from build123d import *

# Parameters (mm, degrees)
F0_W     = 1.5
F0_H     = 30
F1_DEPTH = 3
F0_H_2   = 5
F2_DEPTH = 20
F0_H_3   = 3
F3_DEPTH = 110


with BuildPart() as f1:
    # F0 (on Top) → F1 (new body)
    with BuildSketch(Plane.XY):
        Polygon((12.5, -5), (12.5, 30), (0.75, 30), (0.75, 0), (-0.75, 0), (-0.75, 30), (-12.5, 30), (-12.5, -5), (0, -5), align=None)
        with Locations((0, 15)):
            Rectangle(F0_W, F0_H)
        Polygon((0, -30), (0, -5), (-12.5, -5), (-12.5, -17.5), align=None)
        Polygon((12.5, -17.5), (12.5, -5), (0, -5), (0, -30), align=None)
        Polygon((25, -5), (12.5, -5), (12.5, -17.5), align=None)
        Polygon((-12.5, -17.5), (-12.5, -5), (-25, -5), align=None)
    extrude(amount=F1_DEPTH)

    # F0 (on Top) → F2 (join)
    with BuildSketch(Plane.XY):
        with Locations((0, 32.5)):
            Rectangle(F0_W, F0_H_2)
        with Locations((0, 15)):
            Rectangle(F0_W, F0_H)
        Polygon((0.75, 35), (0.75, 30), (4.75, 35), align=None)
        Polygon((-4.75, 35), (-0.75, 30), (-0.75, 35), align=None)
    extrude(amount=F2_DEPTH)

    # F0 (on Top) → F3 (join)
    with BuildSketch(Plane.XY):
        Polygon((-4.75, 35), (-0.75, 35), (-0.75, 38), (-17, 38), (-17, 35), align=None)
        with Locations((0, 36.5)):
            Rectangle(F0_W, F0_H_3)
        Polygon((0.75, 38), (0.75, 35), (4.75, 35), (17, 35), (17, 38), align=None)
    extrude(amount=F3_DEPTH)


solid = f1.part
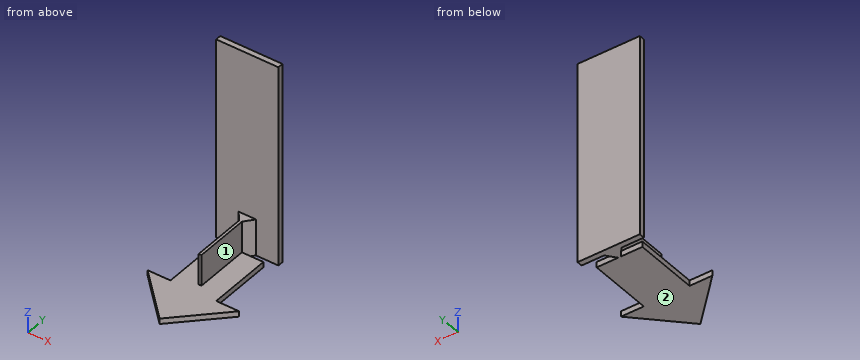
Verification items for the finished model (mm, model axes). Face numbers are marked on the shaded views. A direction names the side the tool comes from. Coordinates: 2 decimals unless noted, no trailing zeros. Write each loop counter-clockwise with the first axis right and the second up, starting at its lowest first coordinate (ties: lowest second). Pieces come first, ordered by that corner, then holes. Notation, with made-up numbers: M 76.25,-38.5 L 83.25,-38.5 A29 ccw 83.25,-13.5 Z; hole C -26,27.5 d10. An arc over 180 degrees is marked long. One line per question, with ' | ' between items.
1) Sectioned sample at B-B on y = 18.5. Record the cut outline in (x, z).
Solutions:
outline: M -12.5,0 L 12.5,0 L 12.5,3 L 0.75,3 L 0.75,20 L -0.75,20 L -0.75,3 L -12.5,3 Z
2) Sectioned sample at C-C on z = 11.5. Record the cut outline in (x, y).
Solutions:
outline: M -17,35 L -4.75,35 L -0.75,30 L -0.75,0 L 0.75,0 L 0.75,30 L 4.75,35 L 17,35 L 17,38 L -17,38 Z
3) Sectioned sample at A-A on x = -7.5. Record the cut outline in (y, z).
Solutions:
outline: M -22.5,0 L 30,0 L 30,3 L -22.5,3 Z; M 35,0 L 38,0 L 38,110 L 35,110 Z
4) Material ranges on L1, parallel to Y at x = -11, z = 21; L2, parallel to Z at x = 9, y = 23; L3, parallel to Z at x = 0, y = 12.5, recorded low to high.
Solutions:
L1: 35 to 38 | L2: 0 to 3 | L3: 0 to 20
5) Depth check by flat-ended pin: pin 1 Ø5 at (y, z) = (17.5, 10) entering from +X; pin 2 Ø7.5 at (x, y) = (-1, 20) entering from +Z; pin 3 Ø3 at (x, y) = (-13.5, 0.5) entering from +Z. Enter the tip coordinate at first touch or a pass-through.
Solutions:
pin 1: x = 0.75 | pin 2: z = 20 | pin 3: z = 3
6) Access from +Z, -Z, +X, -X, +Y, -Y to the whole of each face (thin tool, end or side, straight path). Record for the marked faces 1 and 2.
Solutions:
face 1: +Z, +X, -Y | face 2: -Z, +X, -X, +Y, -Y
7) Sectioned sample at D-D on x = -2. Record the cut outline in (y, z).
Solutions:
outline: M -28,0 L 30,0 L 30,3 L -28,3 Z; M 31.56,0 L 38,0 L 38,110 L 35,110 L 35,20 L 31.56,20 Z
